Can you work these out from the drawing? Everything is in mm from the part's minimum corner. Round coordinates to 2 decimals unless told otherwise and drop trailing zeros. Order: outer loops, then holes, each group sorted by start corner. A loop starts at its lowest first (then second) coordinate and runs counter-clockwise, first axis right, second up. Notation, with made-up numbers: (48, 77.5) -> (85, 77.5) arc R30 ccw to (85, 109.5) -> close; hole circle Ø1 at (52.5, 61). An arc over 180 degrees is marked (long way). One line per item, written item: value.
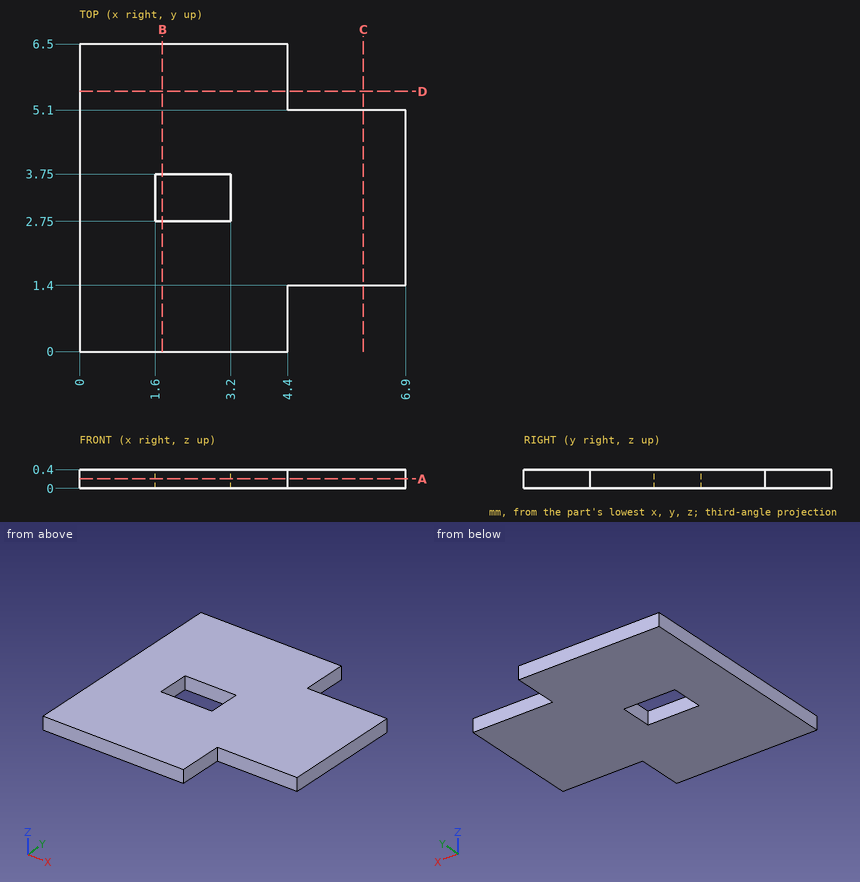
Q1. I need wall thicknesses on line 1 along Y through (x, z) = (2.25, 0.2); line 2 along X through (y, z) = (3.5, 0.1); line 3 along X through (y, z) = (6, 0.35). Which ranges of each line are inside material? Lowest first, please.
Answers:
line 1: 0 to 2.75, 3.75 to 6.5
line 2: 0 to 1.6, 3.2 to 6.9
line 3: 0 to 4.4
Q2. I want a section at B-B on x = 1.75. Write out the boundary of the cut face in (y, z).
Answers:
outline: (0, 0) -> (2.75, 0) -> (2.75, 0.4) -> (0, 0.4) -> close; (3.75, 0) -> (6.5, 0) -> (6.5, 0.4) -> (3.75, 0.4) -> close
Q3. I want a section at D-D on y = 5.5. Write out the boundary of the cut face in (x, z).
Answers:
outline: (0, 0) -> (4.4, 0) -> (4.4, 0.4) -> (0, 0.4) -> close
Q4. I want a section at A-A on z = 0.2. Write out the boundary of the cut face in (x, y).
Answers:
outline: (0, 0) -> (4.4, 0) -> (4.4, 1.4) -> (6.9, 1.4) -> (6.9, 5.1) -> (4.4, 5.1) -> (4.4, 6.5) -> (0, 6.5) -> close; hole (1.6, 2.75) -> (3.2, 2.75) -> (3.2, 3.75) -> (1.6, 3.75) -> close
Q5. For P1, Ø1, axis at x = 4, y = 4, coming from the -Z side, with a flat end and sliding along its axis, tell me the tip position at first contact or that it passes through.
Answers:
P1: z = 0
Q6. I want a section at C-C on x = 6. Write out the boundary of the cut face in (y, z).
Answers:
outline: (1.4, 0) -> (5.1, 0) -> (5.1, 0.4) -> (1.4, 0.4) -> close
